Source: CAD feature listing. Evaluate the final solid. Frame: model axes, mm. A direction names the side the tool comes from. Give positions to 0.01 mm unless a question says otherwise; leave off trailing zeros. Order: outer loops, then holes, each group sorted by start corner. A loop starts at its lowest first (then second) coordinate and runs counter-clockwise, first axis right, second up. Notation, with made-up numbers: M 86,55.5 L 119,55.5 A31 ccw 119,92.5 Z; hole C -18,-19 d4. An arc over 180 degrees is marked long. Answer in a Markdown table with one row per item. Add a question column.
(1) Set-up query: faces 1 (the face through (-29, -3, 0)), 2 (the face through (-53.134, -8, 64)), 3 (the face through (-46, 0, 39)), 4 (the face through (-39, -15.24, 39)). Return all of +Z, -Z, +X, -X, +Y, -Y with unobstructed straight access to the full face (end or side cutting, diameter ignored); none if empty.
(2) Pin query (flat end, axial travel): P1, Ø12, axis at y = -8, z = 65, coming from the -X side; P2, Ø3, axis at y = 7.5, z = 10, coming from the -X side; P3, Ø1.5, axis at x = -39.5, z = 16.5, coming from the +Y side. Return the tip coordinate at first contact, or that it passes through.
(3) Section query A-A, the plane x = -9. Return loops of the section in (y, z), plus the area to 3 significant figures.
(4) Mould query, pull axis Z, two halves, no side actions, for faces 5 (the face through (-7.513, 18.677, 37.793)), 6 (the face through (-14, 6, 76.2)), 7 (the face through (-76.2, -8, 26)), 8 (the face through (-7.513, 55.464, 36.994)). Classes: pulls with the +Z half, pulls with the -Z half, needs draft (parallel to the pull), parting line crosses it, or undercut.
(5) Section query D-D, the plane x = -28. Return loops of the section in (y, z).
(6) Section query C-C, the plane y = 23. Return loops of the section in (x, z).
(7) Material intervals for line 1 along X through (y, z) = (22.5, 12.5); line 2 along Z through (x, y) = (-26.5, -10), sorted ascending.
(8) Section query B-B, the plane z = 53. Return loops of the section in (x, y).
from build123d import *

# Parameters (mm, degrees)
F1_DEPTH = 15.24
F2_R     = 38.1
F3_DEPTH = 15.24
F4_R     = 17.78
F5_DEPTH = 15.24
F6_W     = 38.1
F6_H     = 76.2
F7_DEPTH = 15.24
F8_R     = 17.78
F9_DEPTH = 15.24


with BuildPart() as f1:
    # F0 (on Front) → F1 (new body)
    with BuildSketch(Plane.XZ):
        Polygon((0, 76.2), (-53.134054, 76.2), (-53.134054, 51.589463), (-76.2, 51.589463), (-76.2, 0), (0, 0), align=None)
    extrude(amount=F1_DEPTH)

    # F2 (on Right) → F3 (join)
    with BuildSketch(Plane.YZ):
        with Locations((37.68811, 37.37919)):
            Circle(F2_R)
    extrude(amount=-F3_DEPTH)

    # F4 (on face) → F5 (cut)
    with BuildSketch(Plane.YZ):
        with Locations((37.68811, 37.37919)):
            Circle(F4_R)
    extrude(amount=-F5_DEPTH, mode=Mode.SUBTRACT)

    # F6 (on Right) → F7 (join)
    with BuildSketch(Plane.YZ):
        with Locations((19.05, 38.1)):
            Rectangle(F6_W, F6_H)
    extrude(amount=-F7_DEPTH)

    # F8 (on face) → F9 (cut)
    with BuildSketch(Plane.YZ):
        with Locations((36.452431, 37.37919)):
            Circle(F8_R)
    extrude(amount=-F9_DEPTH, mode=Mode.SUBTRACT)


solid = f1.part
Values follow:
| question | item | result |
|---|---|---|
| 1 | face 1 | -Z, +X, -X, -Y |
| 1 | face 2 | +Z, -X, +Y, -Y |
| 1 | face 3 | +Z, -Z, -X, +Y |
| 1 | face 4 | +Z, -Z, +X, -X, -Y |
| 2 | P1 | stops at x = -53.13 |
| 2 | P2 | stops at x = -15.24 |
| 2 | P3 | stops at y = 0 |
| 3 | outline | M -15.24,0 L 30.31,0 A38.1 ccw long 38.1,75.48 L 38.1,76.2 L -15.24,76.2 Z; hole M 38.1,19.6 A17.78 ccw 38.1,55.15 L 38.1,55.08 A17.78 ccw long 38.1,19.68 Z |
| 3 | area | 5,280 mm² |
| 4 | face 5 | undercut |
| 4 | face 6 | pulls with the +Z half |
| 4 | face 7 | needs draft |
| 4 | face 8 | undercut |
| 5 | outline | M -15.24,0 L 0,0 L 0,76.2 L -15.24,76.2 Z |
| 6 | outline | M -15.24,0 L 0,0 L 0,25.75 L -15.24,25.75 Z; M -15.24,49.01 L 0,49.01 L 0,76.2 L -15.24,76.2 Z |
| 7 | line 1 | x = -15.24 to 0 |
| 7 | line 2 | z = 0 to 76.2 |
| 8 | outline | M -53.13,-15.24 L 0,-15.24 L 0,27.96 L -15.24,27.96 L -15.24,0 L -53.13,0 Z; M -15.24,46.18 L 0,46.18 L 0,72.44 L -15.24,72.44 Z |
